```python
from build123d import *

# Parameters (mm, degrees)
SKETCH1_R                = 0.254
SKETCH1_R_2              = 1.2
BOSS_EXTRUDE1_DEPTH      = 1
SKETCH2_R                = 2.2
SKETCH2_R_2              = 1.2
BOSS_EXTRUDE2_DEPTH      = 2
BOSS_EXTRUDE3_DEPTH      = 1.7018
BOSS_EXTRUDE3_DEPTH_BACK = 2
SKETCH5_R                = 1
CUT_EXTRUDE3_DEPTH       = 2


with BuildPart() as part:
    # Sketch1 → Boss-Extrude1 (new, symmetric)
    with BuildSketch(Plane.XY):
        with BuildLine():
            Line((-5, 5), (-5, -5))
            Line((-5, -5), (45, -5))
            Line((45, -5), (45, -19))
            Line((45, -19), (50, -19))
            Line((50, -19), (50, -17.5))
            ThreePointArc((50, -17.5), (48.5, -16), (50, -14.5))
            Line((50, -14.5), (50, -5))
            Line((50, -5), (50.72, -5))
            Line((50.72, -5), (50.72, 0))
            Line((50.72, 0), (50.72, 5))
            Line((50.72, 5), (50, 5))
            Line((50, 5), (50, 14.5))
            ThreePointArc((50, 14.5), (48.5, 16), (50, 17.5))
            Line((50, 17.5), (50, 19))
            Line((50, 19), (45, 19))
            Line((45, 19), (45, 5))
            Line((45, 5), (-5, 5))
        make_face()
        with Locations((19.22, -2.25)):
            Circle(SKETCH1_R, mode=Mode.SUBTRACT)
        Circle(SKETCH1_R_2, mode=Mode.SUBTRACT)
    extrude(amount=BOSS_EXTRUDE1_DEPTH, both=True)

    # Sketch2 → Boss-Extrude2 (add, symmetric)
    with BuildSketch(Plane.XY):
        Circle(SKETCH2_R)
        Circle(SKETCH2_R_2, mode=Mode.SUBTRACT)
    extrude(amount=BOSS_EXTRUDE2_DEPTH, both=True)

    # Sketch3 → Boss-Extrude3 (add, two sides: drawn at the far end of the back side and taken through both)
    with BuildSketch(Plane(origin=(0, 0, -1), x_dir=(-1, 0, 0), z_dir=(0, 0, -1)).offset(-BOSS_EXTRUDE3_DEPTH_BACK)):
        Polygon((-19.22, -1.696), (-22.22, -1.696), (-22.22, -13.696), (-16.22, -13.696), (-16.22, -12.696), (-16.22, -11.696), (-16.22, -9.062), (-16.22, -1.696), align=None)
    extrude(amount=BOSS_EXTRUDE3_DEPTH + BOSS_EXTRUDE3_DEPTH_BACK)

    # Sketch5 → Cut-Extrude3 (cut)
    with BuildSketch(Plane(origin=(0, 0, -2.7018), x_dir=(-1, 0, 0), z_dir=(0, 0, -1))):
        with Locations((-19.22, -4.696)):
            Circle(SKETCH5_R)
    extrude(amount=-CUT_EXTRUDE3_DEPTH, mode=Mode.SUBTRACT)


solid = part.part
```
The listing builds one solid part. Answer for the finished solid, in the listing's coordinates (mm). A direction names the side the tool comes from. Round coordinates to 2 decimals unless told otherwise and drop trailing zeros. Loops run counter-clockwise (first coordinate to the right, second up) from the corner with the lowest first, then second, coordinate; pieces in that order, holes last. Notation, with made-up numbers: (-25, 65.5) - (2, 65.5) arc R14 cw to (2, 73.5) - close; hole circle Ø2 at (34.25, 14). An arc over 180 degrees is marked (long way). Return JSON: item names as keys, results as strings. Group by question number.
1. The mould has two halves that part along X. Classify faces 6 (the flat face through (33, -5, 0)), 7 (the cylindrical face through (0.65, 1.01, -0.03)), 8 (the flat face through (19, -1.696, -2)), 9 (the cylindrical face through (48.5, -16, 0)): pulls with the +X half, pulls with the -X half, needs draft (parallel to the pull), parting line crosses it, or undercut.
2. The part is cut by section A-A on z = 0.05. Determine the outline of the cut face in (x, y).
3. The part is cut by section D-D on x = 19.22. Determine the outline of the cut face in (y, z), then the cut area to 3 significant figures.
4. Which of the six approach directions +Z, -Z, +X, -X, +Y, -Y give full straight-line access (tool end or side, diameter ignored) to faces 1 (the flat face through (50, -10, 0)), 2 (the flat face through (45, -12, 0)), 3 (the flat face through (50, 10, 0)), 4 (the cylindrical face through (20.22, -4.65, -1.72)), 5 (the flat face through (5, -5, 0))?
5. Each of these flat-tipped pins is pushed along its axis until it touches: P1, Ø11.5, axis at x = 25.5, y = 9, coming from the -Z side; P2, Ø2, axis at x = 17, y = -10.5, coming from the +Z side; P3, Ø0.9, axis at x = 18.5, z = -2, coming from the +Y side. Where does it stop, or does it pass through?
6. Consider probe 1 along Y at (x, z) = (0, -0.3); probe 2 along X at (y, z) = (-7, -0.3); probe 3 along Y at (x, z) = (0, -1.75). Determine where each line is inside the solid, lowest interval first.
7. The part is cut by section B-B on x = 0. Determine the outline of the cut face in (y, z), then the cut area to 3 significant figures.
8. The part is cut by section C-C on y = -7. Determine the outline of the cut face in (x, z).
Resolved:
{
 "1": {"face 6": "undercut", "face 7": "undercut", "face 8": "needs draft", "face 9": "pulls with the +X half"},
 "2": {"outline": "(-5, -5) - (16.22, -5) - (16.22, -13.7) - (22.22, -13.7) - (22.22, -5) - (45, -5) - (45, -19) - (50, -19) - (50, -17.5) arc R1.5 cw to (50, -14.5) - (50, -5) - (50.72, -5) - (50.72, 5) - (50, 5) - (50, 14.5) arc R1.5 cw to (50, 17.5) - (50, 19) - (45, 19) - (45, 5) - (-5, 5) - close; hole circle Ø2.4 at (0, 0)"},
 "3": {"outline": "(-13.7, -2.7) - (-5.7, -2.7) - (-5.7, -0.7) - (-3.7, -0.7) - (-3.7, -2.7) - (-1.7, -2.7) - (-1.7, -1) - (5, -1) - (5, 1) - (-13.7, 1) - close", "area": "53.8 mm²"},
 "4": {"face 1": "+Z, -Z, +X, -Y", "face 2": "+Z, -Z, -Y", "face 3": "+Z, -Z, +X, +Y", "face 4": "-Z", "face 5": "+Z, -Z, -X, -Y"},
 "5": {"P1": "stops at z = -1", "P2": "stops at z = 1", "P3": "stops at y = -1.7"},
 "6": {"probe 1": "y = -5 to -1.2, 1.2 to 5", "probe 2": "x = 16.22 to 22.22, 45 to 50", "probe 3": "y = -2.2 to -1.2, 1.2 to 2.2"},
 "7": {"outline": "(-5, -1) - (-2.2, -1) - (-2.2, -2) - (-1.2, -2) - (-1.2, 2) - (-2.2, 2) - (-2.2, 1) - (-5, 1) - close; (1.2, -2) - (2.2, -2) - (2.2, -1) - (5, -1) - (5, 1) - (2.2, 1) - (2.2, 2) - (1.2, 2) - close", "area": "19.2 mm²"},
 "8": {"outline": "(16.22, -2.7) - (22.22, -2.7) - (22.22, 1) - (16.22, 1) - close; (45, -1) - (50, -1) - (50, 1) - (45, 1) - close"}
}
